from build123d import *

# Parameters (mm, degrees)
SKETCH1_R           = 4.7625
SKETCH1_R_2         = 2.38125
BOSS_EXTRUDE1_DEPTH = 3.175


with BuildPart() as part:
    # Sketch1 → Boss-Extrude1 (new body)
    # profile 1 of 3: a face of its own
    with BuildSketch(Plane.XY):
        with BuildLine():
            Line((-4.7625, 12.7), (-4.7625, 0))
            ThreePointArc((-4.7625, 0), (0, 4.7625), (4.7625, 0))
            Line((4.7625, 0), (4.7625, 12.7))
            ThreePointArc((4.7625, 12.7), (0, 7.9375), (-4.7625, 12.7))
        make_face()
    # profile 2 of 3: a face of its own
    with BuildSketch(Plane.XY):
        with Locations((0, 12.7)):
            Circle(SKETCH1_R)
        with Locations((0, 12.7)):
            Circle(SKETCH1_R_2, mode=Mode.SUBTRACT)
    # profile 3 of 3: a face of its own
    with BuildSketch(Plane.XY):
        Circle(SKETCH1_R)
        Circle(SKETCH1_R_2, mode=Mode.SUBTRACT)
    extrude(amount=BOSS_EXTRUDE1_DEPTH)


solid = part.part
Could you check a few things on this model? Use its own coordinates, in mm. Give positions to 0.01 mm unless a question says otherwise; leave off trailing zeros. Order: outer loops, then holes, each group sorted by start corner. A loop starts at its lowest first (then second) coordinate and runs counter-clockwise, first axis right, second up.
Item 1: I'm going to push flat-ended pins straight in: pin 1 (1.5 mm diameter, centred on x = -1, z = 0.5, fed in from -Y); pin 2 (4.5 mm diameter, centred on x = 0, y = 0, fed in from -Z); pin 3 (1 mm diameter, centred on x = -2.5, z = 0.5, fed in from -Y). Where does each tip first touch, or does it pass through?
Item 2: If we section it at D-D, the plane y = -1: Write out the boundary of the cut face in (x, z) (3 decimals), plus the area to 3 significant figures.
Item 3: If we mould it in two halves opening along X, with no side actions, what happens to faces 1 (the face through (-0.31, 15.06, 1.57)), 2 (the face through (0, 7, 3.175)), 3 (the face through (4.762, 6, 2)), 4 (the face through (-0.1, -4.76, 1.57))? For each: pulls with the +X half, pulls with the -X half, needs draft (parallel to the pull), parting line crosses it, or undercut.
Item 4: If we section it at C-C, the plane y = 14: Write out the boundary of the cut face in (x, z) (3 decimals).
Item 5: If we section it at B-B, the plane z = 2.25: Write out the boundary of the cut face in (x, y) (1 decimal).
Item 6: If we section it at A-A, the plane x = 0: Write out the boundary of the cut face in (y, z) (1 decimal), plus the area to 3 significant figures.
Item 7: I need wall thicknesses on line 1 (Y direction, x = 0, z = 2.4); line 2 (Y direction, x = -2, z = 2.15); line 3 (X direction, y = 14.75, z = 0.65). Which ranges of each line are inside material? Lowest first, please.
Values:
1. pin 1: stops at y = -4.76
1. pin 2: passes through
1. pin 3: stops at y = -4.32
2. outline: (-4.656, 0) - (-2.161, 0) - (-2.161, 3.175) - (-4.656, 3.175) - close; (2.161, 0) - (4.656, 0) - (4.656, 3.175) - (2.161, 3.175) - close
2. area: 15.8 mm2
3. face 1: undercut
3. face 2: needs draft
3. face 3: pulls with the +X half
3. face 4: parting line crosses it
4. outline: (-4.582, 0) - (-1.995, 0) - (-1.995, 3.175) - (-4.582, 3.175) - close; (1.995, 0) - (4.582, 0) - (4.582, 3.175) - (1.995, 3.175) - close
5. outline: (-4.8, 0) arc R4.8 ccw to (4.8, 0) - (4.8, 12.7) arc R4.8 ccw to (-4.8, 12.7) - close; hole circle Ø4.8 at (0, 0); hole circle Ø4.8 at (0, 12.7)
6. outline: (-4.8, 0) - (-2.4, 0) - (-2.4, 3.2) - (-4.8, 3.2) - close; (2.4, 0) - (10.3, 0) - (10.3, 3.2) - (2.4, 3.2) - close; (15.1, 0) - (17.5, 0) - (17.5, 3.2) - (15.1, 3.2) - close
6. area: 40.3 mm2
7. line 1: y = -4.76 to -2.38, 2.38 to 10.32, 15.08 to 17.46
7. line 2: y = -4.32 to -1.29, 1.29 to 11.41, 13.99 to 17.02
7. line 3: x = -4.3 to -1.21, 1.21 to 4.3
